For this review, take the finished solid that the model builds, in its own axes (mm). Face numbers are marked on the shaded views. A direction names the side the tool comes from. Give positions to 0.01 mm unless a question says otherwise; leave off trailing zeros. Write each loop counter-clockwise with the first axis right and the second up, starting at its lowest first coordinate (ties: lowest second). Pieces come first, ordered by that corner, then holes. Notation, with made-up numbers: (-29, 1) -> (28, 1) arc R21 cw to (28, 9) -> close; hole circle Ø3 at (-10, 24). An arc over 180 degrees is marked (long way). Answer as CSV lines item,"result".
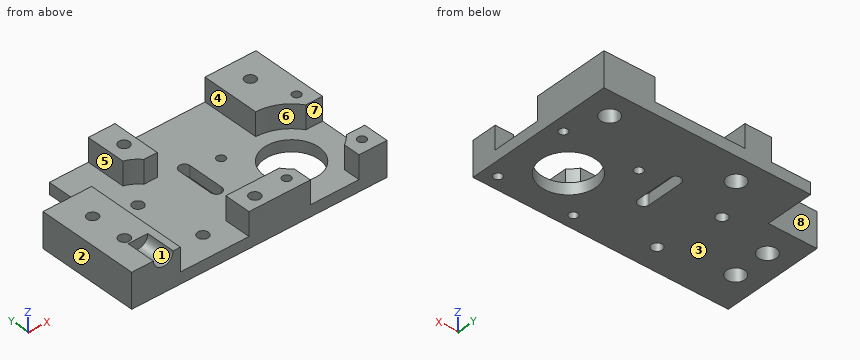
```python
from build123d import *

# Parameters (mm, degrees)
SKETCH_R        = 2.25
SKETCH_R_2      = 11.25
SKETCH_R_3      = 1.75
PAD_DEPTH       = 14.3
POCKET_DEPTH    = 9.6
SKETCH004_R     = 2.25
POCKET003_DEPTH = 10
SKETCH005_R     = 4.05
POCKET004_DEPTH = 12
SKETCH006_R     = 3.75
POCKET005_DEPTH = 9.2


with BuildPart() as part:
    # Sketch → Pad (new body)
    with BuildSketch(Plane.XY):
        Polygon((0, 0), (105, 0), (105, 62), (20, 62), (20, 42), (0, 42), align=None)
        with Locations((38, 10)):
            Circle(SKETCH_R, mode=Mode.SUBTRACT)
        with Locations((33, 35)):
            Circle(SKETCH_R, mode=Mode.SUBTRACT)
        with Locations((84, 21)):
            Circle(SKETCH_R_2, mode=Mode.SUBTRACT)
        with Locations((68.5, 36.5)):
            Circle(SKETCH_R_3, mode=Mode.SUBTRACT)
        with Locations((99.5, 36.5)):
            Circle(SKETCH_R_3, mode=Mode.SUBTRACT)
        with Locations((68.5, 5.5)):
            Circle(SKETCH_R_3, mode=Mode.SUBTRACT)
        with Locations((99.5, 5.5)):
            Circle(SKETCH_R_3, mode=Mode.SUBTRACT)
        with Locations((10, 30)):
            Circle(SKETCH_R, mode=Mode.SUBTRACT)
        with Locations((10, 15)):
            Circle(SKETCH_R, mode=Mode.SUBTRACT)
        with Locations((42, 52)):
            Circle(SKETCH_R, mode=Mode.SUBTRACT)
        with Locations((94, 52)):
            Circle(SKETCH_R, mode=Mode.SUBTRACT)
        with BuildLine():
            Line((58.75, 25), (58.75, 39.999999))
            ThreePointArc((58.75, 39.999999), (56.5, 42.25), (54.25, 39.999998))
            Line((54.25, 25.000001), (54.25, 39.999998))
            ThreePointArc((54.25, 25.000001), (56.5, 22.75), (58.75, 25))
        make_face(mode=Mode.SUBTRACT)
    extrude(amount=PAD_DEPTH)

    # Sketch001 → Pocket (cut)
    with BuildSketch(Plane.XY.offset(14.3)):
        with BuildLine():
            ThreePointArc((41.485277, 42), (39.015593, 44.209375), (35.999996, 45.583005))
            Line((35.999996, 67), (35.999996, 45.583005))
            Line((20, 67), (35.999996, 67))
            Line((20, -1), (20, 67))
            Line((20, -1), (48.252269, -1))
            Line((48.252269, 11), (48.252269, -1))
            Line((48.252269, 11), (70.252269, 11))
            ThreePointArc((70.252269, 11), (71.759618, 9.202833), (73.499996, 7.630258))
            Line((73.499996, 7.630258), (73.499996, -1))
            Line((73.499996, -1), (93.499996, -1))
            Line((93.499996, -1), (93.499996, 6.902128))
            ThreePointArc((93.499996, 6.902128), (95.574295, 8.548671), (97.367695, 10.497399))
            Line((105.499996, 10.497399), (97.367695, 10.497399))
            Line((105.499996, 30.497399), (105.499996, 10.497399))
            Line((98.099621, 30.497399), (105.499996, 30.497399))
            ThreePointArc((98.099621, 30.497399), (91.98574, 36.007594), (83.999996, 38))
            Line((83.999996, 38), (83.999996, 67))
            Line((83.999996, 67), (46.999996, 67))
            Line((46.999996, 67), (46.999996, 42))
            Line((41.485277, 42), (46.999996, 42))
        make_face()
    extrude(amount=-POCKET_DEPTH, mode=Mode.SUBTRACT)

    # Sketch004 → Pocket003 (cut)
    with BuildSketch(Plane.XY.offset(14.3)):
        with Locations((55, 5)):
            Circle(SKETCH004_R)
    extrude(amount=-POCKET003_DEPTH, mode=Mode.SUBTRACT)

    # Sketch005 → Pocket004 (cut)
    with BuildSketch(Plane.XZ):
        with Locations((13, 14.3)):
            Circle(SKETCH005_R)
    extrude(amount=-POCKET004_DEPTH, mode=Mode.SUBTRACT)

    # Sketch006 → Pocket005 (cut)
    with BuildSketch(Plane(origin=(0, 0, 0), x_dir=(1, 0, 0), z_dir=(0, 0, -1))):
        with Locations((10, -15)):
            Circle(SKETCH006_R)
        with Locations((10, -30)):
            Circle(SKETCH006_R)
        with Locations((42, -52)):
            Circle(SKETCH006_R)
        with Locations((94, -52)):
            Circle(SKETCH006_R)
    extrude(amount=-POCKET005_DEPTH, mode=Mode.SUBTRACT)


solid = part.part
```
Q1. To check wall thickness, follow probe 1 along Y at (x, z) = (99.5, 8.75); probe 2 along Y at (x, z) = (13, 6.75); probe 3 along X at (y, z) = (52, 12.1). State the ranges of each line that lie inside material, in increasing order. Write a range as [from, to].
Answer block:
probe 1,"y = [0, 3.75], [7.25, 10.5], [30.5, 34.75], [38.25, 62]"
probe 2,"y = [0, 12.75], [17.25, 27.75], [32.25, 42]"
probe 3,"x = [36, 39.75], [44.25, 47], [84, 91.75], [96.25, 105]"
Q2. For the marked faces 4, 5, 6, 7 and 8, list the 3-axis set-ups (+Z, -Z, +X, -X, +Y, -Y) from which the entire face can be reached by the end or side of a thin tool; tool diameter is ignored.
Answer block:
face 4,"+Z, +Y, -Y"
face 5,"+Z, -X, +Y, -Y"
face 6,"+Z"
face 7,"+Z, +X"
face 8,"+Z, -Z, -X, +Y"
Q3. Add section A-A (z = 7.5). State how many separate pieces and enclosed holes the cut face has, plus the area to 3 significant figures.
Answer block:
separate pieces,"5"
enclosed holes,"8"
area,"1,800 mm2"
Q4. Draft analysis for pull direction X (two halves, no side actions). For the marked faces 1, 2 and 3, state which applies: released by +X, released by -X, zero draft, split by the parting line, or undercut.
Answer block:
face 1,"undercut"
face 2,"released by -X"
face 3,"zero draft"
Q5. Clearance check with flat-ended pins moving along their axes: pin 1 (1.5 mm diameter, centred on x = 64, y = 28, fed in from +Z); pin 2 (2 mm diameter, centred on x = 41.5, y = 53.5, fed in from -Z); pin 3 (5 mm diameter, centred on y = 52.5, z = 10, fed in from -X); pin 4 (2 mm diameter, centred on x = 99.5, y = 36.5, fed in from +Z). State where each tip first meets the part, or that it passes through.
Answer block:
pin 1,"stops at z = 4.7"
pin 2,"stops at z = 9.2"
pin 3,"stops at x = 36"
pin 4,"passes through"
Q6. Add section C-C (y = 21). Write out the cut boundary in (x, z).
Answer block:
outline,"(0, 0) -> (72.75, 0) -> (72.75, 4.7) -> (20, 4.7) -> (20, 14.3) -> (0, 14.3) -> close; (95.25, 0) -> (105, 0) -> (105, 4.7) -> (95.25, 4.7) -> close"
Q7. Add section B-B (x = 68.5). Write out the cut boundary in (y, z).
Answer block:
outline,"(0, 0) -> (3.75, 0) -> (3.75, 14.3) -> (0, 14.3) -> close; (7.25, 0) -> (34.75, 0) -> (34.75, 4.7) -> (11, 4.7) -> (11, 14.3) -> (7.25, 14.3) -> close; (38.25, 0) -> (62, 0) -> (62, 4.7) -> (38.25, 4.7) -> close"
